Can you work these out from the model? Positions are in its coordinate system, mm. A direction names the side the tool comes from. Round coordinates to 2 decimals unless told otherwise and drop trailing zeros. Loops run counter-clockwise (first coordinate to the right, second up) from the corner with the lowest first, then second, coordinate; pieces in that order, holes last.
(1) I want a section at D-D on x = -10.5. Write out the boundary of the cut face in (y, z).
(2) I want a section at C-C on z = 19. Write out the boundary of the cut face in (x, y), plus the area to 3 significant figures.
(3) If I drill on line 1 along X through (y, z) = (15, 7.5); line 2 along Y through (x, z) = (41.9, 26.4); line 3 along Y through (x, z) = (-10.5, -1), over which ranges is the centre line in solid material (lowest first)?
(4) Which directions (+Z, -Z, +X, -X, +Y, -Y) give clear straight access to the entire face, cutting with the end or side of a thin tool? Please do faces 1 (the face through (-37, 26.4, 9)), 2 (the face through (-42, 0, 4)), 3 (the face through (-32, 7, 3)).
(5) I want a section at B-B on z = 10.5. Give the number of separate pieces and of enclosed holes in the cut face, plus the area to 3 significant figures.
(6) Will these pins go through, and if not, where does the flat tip stop? pin 1 Ø1 at (x, y) = (-31, -12.5) entering from +Z; pin 2 Ø12 at (x, y) = (-18.5, 36) entering from +Z; pin 3 Ø5.5 at (x, z) = (-32.5, 15.5) entering from +Y; pin 4 Ø9.5 at (x, z) = (-27.5, 20.5) entering from -Y.
(7) Thinking about a two-plate mould opening in Y: for faces 4 (the face through (47.69, 15.02, -1.48)), 5 (the face through (16.5, 7, 7)), 6 (the face through (0, 7, 0)), 7 (the face through (-37, -12.6, 9)), which applies, released by +Y, released by -Y, zero draft, split by the parting line, or undercut?
(8) I want a section at A-A on x = 0. Write out the boundary of the cut face in (y, z).
from build123d import *

# Parameters (mm, degrees)
EXTRUDE_START            = 26.4
EXTRUDE_3_DEPTH          = 39
SHELL_2_T                = -3
SKETCH_7_R               = 6.75
SKETCH_7_R_2             = 1.4
CUT_EXTRUDE_5_DEPTH      = 47.496881616
SKETCH_1_R               = 50
EXTRUDE_1_DEPTH          = 3
SKETCH_9_W               = 33
SKETCH_9_H               = 38.7
SKETCH_9_W_2             = 27
SKETCH_9_H_2             = 32.7
EXTRUDE_5_DEPTH          = 15
CUT_EXTRUDE_8_DEPTH      = 79.89866919
CUT_EXTRUDE_8_DEPTH_BACK = 79.89866919
SKETCH_8_R               = 1.4
SKETCH_8_R_2             = 6.5


# Read off the part's stored shape, not the designer's step: ﾐﾗｰ1
with BuildPart() as part:
    # ｽｹｯﾁ5 → ﾎﾞｽ - 押し出し3 (new body)
    with BuildSketch(Plane(origin=(0, 0, 0), x_dir=(1, 0, 0), z_dir=(0, 1, 0)).offset(EXTRUDE_START)):
        Polygon((-44, -32), (-44, 0), (-20, 0), align=None)
    extrude(amount=-EXTRUDE_3_DEPTH)

    # ｼｪﾙ2
    shell_2_openings = [part.faces().sort_by_distance(p)[0] for p in [
        (-32, 6.9, 16),
    ]]
    offset(amount=SHELL_2_T, openings=shell_2_openings, kind=Kind.INTERSECTION)

    # ｽｹｯﾁ7 → ｶｯﾄ - 押し出し5 (cut, through all)
    with BuildSketch(Plane(origin=(-41, 0, 0), x_dir=(0, 0, -1), z_dir=(1, 0, 0))):
        with Locations((-15.9, 0)):
            Circle(SKETCH_7_R)
        with Locations((-26.4, 0)):
            Circle(SKETCH_7_R_2)
        with Locations((-5.4, 0)):
            Circle(SKETCH_7_R_2)
        with Locations((-5.4, 21)):
            Circle(SKETCH_7_R_2)
        with Locations((-26.4, 21)):
            Circle(SKETCH_7_R_2)
    extrude(amount=-CUT_EXTRUDE_5_DEPTH, mode=Mode.SUBTRACT)

    # ｽｹｯﾁ1 → ﾎﾞｽ - 押し出し1 (add)
    with BuildSketch(Plane.XY):
        Circle(SKETCH_1_R)
    extrude(amount=-EXTRUDE_1_DEPTH)

    # ﾐﾗｰ1: part across plane


with BuildPart() as part_1:
    add(part.part)
    add(part.part.mirror(Plane(origin=(0, 0, 0), x_dir=(0, 0, 1), z_dir=(1, 0, 0))))

    # ｽｹｯﾁ9 → ﾎﾞｽ - 押し出し5 (add)
    with BuildSketch(Plane.XY):
        with Locations((0, 6.95)):
            Rectangle(SKETCH_9_W, SKETCH_9_H)
        with Locations((0, 6.95)):
            Rectangle(SKETCH_9_W_2, SKETCH_9_H_2, mode=Mode.SUBTRACT)
    extrude(amount=EXTRUDE_5_DEPTH)

    # ｽｹｯﾁ8 → ｶｯﾄ - 押し出し8 (cut, two sides: drawn at the far end of the back side and taken through both)
    with BuildSketch(Plane(origin=(0, 0, -3), x_dir=(-1, 0, 0), z_dir=(0, 0, -1)).offset(-CUT_EXTRUDE_8_DEPTH_BACK)):
        with Locations(Location((-10.5, 21, 0), (0, 0, 180))):
            Circle(SKETCH_8_R)
        with Locations(Location((10.5, 21, 0), (0, 0, 180))):
            Circle(SKETCH_8_R)
        with Locations(Location((-10.5, 0, 0), (0, 0, 180))):
            Circle(SKETCH_8_R)
        with Locations(Location((10.5, 0, 0), (0, 0, 180))):
            Circle(SKETCH_8_R)
        with Locations(Location((0, 0, 0), (0, 0, 180))):
            Circle(SKETCH_8_R_2)
    extrude(amount=CUT_EXTRUDE_8_DEPTH + CUT_EXTRUDE_8_DEPTH_BACK, mode=Mode.SUBTRACT)


solid = part_1.part
Filled sheet:
1. outline: (-48.89, -3) - (-1.4, -3) - (-1.4, 0) - (-9.4, 0) - (-9.4, 15) - (-12.4, 15) - (-12.4, 0) - (-48.89, 0) - close; (1.4, -3) - (19.6, -3) - (19.6, 0) - (1.4, 0) - close; (22.4, -3) - (48.89, -3) - (48.89, 0) - (26.3, 0) - (26.3, 15) - (23.3, 15) - (23.3, 0) - (22.4, 0) - close
2. outline: (-44, -12.6) - (-34.25, -12.6) - (-34.25, -9.6) - (-41, -9.6) - (-41, -6) - (-44, -6) - close; (-44, 6) - (-41, 6) - (-41, 23.4) - (-34.25, 23.4) - (-34.25, 26.4) - (-44, 26.4) - close; (34.25, -12.6) - (44, -12.6) - (44, -6) - (41, -6) - (41, -9.6) - (34.25, -9.6) - close; (34.25, 23.4) - (41, 23.4) - (41, 6) - (44, 6) - (44, 26.4) - (34.25, 26.4) - close
2. area: 243 mm2
3. line 1: x = -44 to -41, -16.5 to -13.5, 13.5 to 16.5, 41 to 44
3. line 2: y = -12.6 to -1.4, 1.4 to 19.6, 22.4 to 26.4
3. line 3: y = -48.89 to -1.4, 1.4 to 19.6, 22.4 to 48.89
4. face 1: +Z, +X, -X, +Y
4. face 2: -X
4. face 3: +Z
5. separate pieces: 5
5. enclosed holes: 1
5. area: 737 mm2
6. pin 1: stops at z = 15.33
6. pin 2: stops at z = 0
6. pin 3: stops at y = 26.4
6. pin 4: passes through
7. face 4: split by the parting line
7. face 5: zero draft
7. face 6: undercut
7. face 7: released by -Y
8. outline: (-50, -3) - (-6.5, -3) - (-6.5, 0) - (-9.4, 0) - (-9.4, 15) - (-12.4, 15) - (-12.4, 0) - (-50, 0) - close; (6.5, -3) - (50, -3) - (50, 0) - (26.3, 0) - (26.3, 15) - (23.3, 15) - (23.3, 0) - (6.5, 0) - close
